```python
from build123d import *

# Parameters (mm, degrees)
SKETCH_1_W          = 280
SKETCH_1_H          = 60
EXTRUDE_1_DEPTH     = 4
HOLE_WIZARD_M4_1_D  = 3.3
SKETCH_10_W         = 3
SKETCH_10_H         = 60
EXTRUDE_4_DEPTH     = 95
EXTRUDE_8_DEPTH     = 60
SKETCH_14_W         = 75
SKETCH_14_H         = 45
EXTRUDE_10_DEPTH    = 10
SHELL_START         = -12
SHELL_1_OUTLINE_W   = 69
SHELL_1_OUTLINE_H   = 7
SHELL_1_DEPTH       = 42
SHELL_START_2       = -27
SHELL_1_2_DEPTH     = 15
CUT_EXTRUDE_2_REACH = 309.898
CUT_EXTRUDE_3_REACH = 184.211


# Read off the part's stored shape, not the designer's step: 抽壳1
with BuildPart() as part:
    # 草图1 → 凸台-拉伸1 (new body)
    with BuildSketch(Plane(origin=(0, 0, 0), x_dir=(0, 0, -1), z_dir=(1, 0, 0))):
        Rectangle(SKETCH_1_W, SKETCH_1_H)
    extrude(amount=EXTRUDE_1_DEPTH)

    # M4 螺纹孔1 (through all)
    with Locations(Plane(origin=(4, 20, -129), x_dir=(0, 0, 1), z_dir=(1, 0, 0))):
        with Locations((0, 0), (28, 0), (28, 40), (0, 40)):
            Hole(HOLE_WIZARD_M4_1_D / 2)

    # 草图10 → 凸台-拉伸4 (add)
    with BuildSketch(Plane(origin=(4, 0, 0), x_dir=(0, 0, -1), z_dir=(1, 0, 0))):
        with Locations((-138.5, 0)):
            Rectangle(SKETCH_10_W, SKETCH_10_H)
    extrude(amount=EXTRUDE_4_DEPTH)

    # 草图11 → 凸台-拉伸8 (add)
    with BuildSketch(Plane(origin=(0, 30, 0), x_dir=(1, 0, 0), z_dir=(0, 1, 0))):
        Polygon((4, -127), (14, -137), (4, -137), align=None)
    extrude(amount=-EXTRUDE_8_DEPTH)

    # 草图14 → 凸台-拉伸10 (add)
    with BuildSketch(Plane.XY.offset(140)):
        with Locations((61.5, 7.5)):
            Rectangle(SKETCH_14_W, SKETCH_14_H)
    extrude(amount=EXTRUDE_10_DEPTH)

    # 抽壳1 outline → 抽壳1 (cut)
    with BuildSketch(Plane(origin=(0, 0, 0), x_dir=(1, 0, 0), z_dir=(0, 1, 0)).offset(SHELL_START)):
        with Locations((61.5, -143.5)):
            Rectangle(SHELL_1_OUTLINE_W, SHELL_1_OUTLINE_H)
        Polygon((3, -137), (9.757359313, -137), (3, -130.242640687), align=None)
    extrude(amount=SHELL_1_DEPTH, mode=Mode.SUBTRACT)

    # Shell 1 2 outline → Shell 1 2 (cut)
    with BuildSketch(Plane(origin=(0, 0, 0), x_dir=(1, 0, 0), z_dir=(0, 1, 0)).offset(SHELL_START_2)):
        Polygon((3, -137), (9.757359313, -137), (3, -130.242640687), align=None)
    extrude(amount=SHELL_1_2_DEPTH, mode=Mode.SUBTRACT)

    # 切除-拉伸2: up to this face of the body (flat: up to its plane)
    cut_extrude_2_end = Plane(part.part.faces().sort_by_distance((56.5, 0, 137))[0])
    # 草图15 → 切除-拉伸2 (cut, up to the picked face)
    with BuildSketch(Plane.XY.offset(150), mode=Mode.PRIVATE) as cut_extrude_2_sk1:
        Polygon((61.5, 30), (29, 30), (29, 5), (44, -10), (61.5, -10), align=None)
    cut_extrude_2_tool1 = split(extrude(cut_extrude_2_sk1.sketch, amount=-CUT_EXTRUDE_2_REACH, mode=Mode.PRIVATE), bisect_by=cut_extrude_2_end, keep=Keep.BOTH, mode=Mode.PRIVATE)
    # 草图15 → 切除-拉伸2 (cut, up to the picked face)
    with BuildSketch(Plane.XY.offset(150), mode=Mode.PRIVATE) as cut_extrude_2_sk2:
        Polygon((94, 30), (61.5, 30), (61.5, -10), (79, -10), (94, 5), align=None)
    cut_extrude_2_tool2 = split(extrude(cut_extrude_2_sk2.sketch, amount=-CUT_EXTRUDE_2_REACH, mode=Mode.PRIVATE), bisect_by=cut_extrude_2_end, keep=Keep.BOTH, mode=Mode.PRIVATE)
    add(cut_extrude_2_tool1.solids().sort_by(Axis((46.315789, 11.421053, 150), (0, 0, -1)))[0], mode=Mode.SUBTRACT)
    add(cut_extrude_2_tool2.solids().sort_by(Axis((76.684211, 11.421053, 150), (0, 0, -1)))[0], mode=Mode.SUBTRACT)

    # 草图16 → 切除-拉伸3 (cut, up to next)
    with BuildSketch(Plane.ZY, mode=Mode.PRIVATE) as cut_extrude_3_sk1:
        with BuildLine():
            Line((-76, 24), (120, 24))
            ThreePointArc((120, 24), (127.071067812, 21.071067812), (130, 14))
            Line((130, 14), (130, -14))
            ThreePointArc((130, -14), (127.071067812, -21.071067812), (120, -24))
            Line((120, -24), (-76, -24))
            ThreePointArc((-76, -24), (-83.071067812, -21.071067812), (-86, -14))
            Line((-86, -14), (-86, 14))
            ThreePointArc((-86, 14), (-83.071067812, 21.071067812), (-76, 24))
        make_face()
    cut_extrude_3_tool1 = extrude(cut_extrude_3_sk1.sketch, amount=-CUT_EXTRUDE_3_REACH, mode=Mode.PRIVATE) & part.part
    add(cut_extrude_3_tool1.solids().sort_by_distance((0, 0, 22))[0], mode=Mode.SUBTRACT)


solid = part.part
```
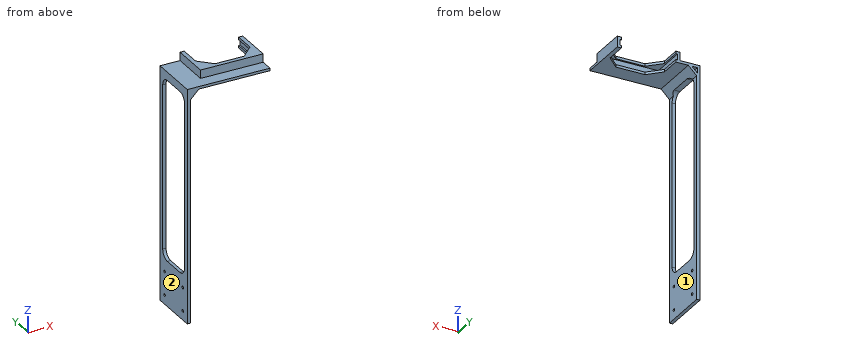
The listing builds one solid part. Answer for the finished solid, in the listing's coordinates (mm). Face numbers are marked on the shaded views. A direction names the side the tool comes from. Coordinates: 2 decimals unless noted, no trailing zeros. Loops run counter-clockwise (first coordinate to the right, second up) from the corner with the lowest first, then second, coordinate; pieces in that order, holes last. Notation, with made-up numbers: (64, 53.5) - (84, 53.5) arc R30 cw to (84, 76.5) - close; hole circle Ø6 at (-17.75, -10). An arc over 180 degrees is marked (long way). Write item = value, one per line.
1) Section C-C (x = 51.5) is taken. Determine the outline of the cut face in (y, z), plus the area to 3 significant figures.
Responses:
outline = (-30, 137) - (-10, 137) - (-10, 140) - (-12, 140) - (-12, 147) - (-10, 147) - (-10, 150) - (-15, 150) - (-15, 140) - (-30, 140) - close
area = 96.0 mm^2
2) Section B-B (z = -70) is taken. Determine the outline of the cut face in (x, y).
Responses:
outline = (0, -30) - (4, -30) - (4, -24) - (0, -24) - close; (0, 24) - (4, 24) - (4, 30) - (0, 30) - close
3) Find the intervals of material crossed by line 1 along Y through (x, z) = (2.55, -129); line 2 along Z through (x, y) = (1.5, -20); line 3 along Z through (x, y) = (29, -2), in increasing order.
Responses:
line_1 = -30 to -21.65, -18.35 to 18.35, 21.65 to 30
line_2 = -140 to -130.65, -127.35 to -102.65, -99.35 to -84, 128 to 140
line_3 = 137 to 140, 147 to 150
4) Each of these flat-tipped pins is pushed along its axis until it touches: P1, Ø5.5, axis at x = 7, z = 134.5, coming from the +Y side; P2, Ø0.9, axis at x = 54, z = 148, coming from the +Y side; P3, Ø8, axis at x = 72, z = 144.5, coming from the -Y side; P4, Ø5.5, axis at y = -4.5, z = 133.5, coming from the +X side. Where does it stop, or does it pass through?
Responses:
P1 = 30
P2 = -10
P3 = -15
P4 = 13.25
5) Section A-A (y = -5) is taken. Determine the outline of the cut face in (x, z).
Responses:
outline = (0, -140) - (4, -140) - (4, -86) - (0, -86) - close; (0, 130) - (7, 130) - (14, 137) - (39, 137) - (39, 140) - (27, 140) - (27, 147) - (39, 147) - (39, 150) - (24, 150) - (24, 140) - (0, 140) - close; (84, 137) - (99, 137) - (99, 150) - (84, 150) - (84, 147) - (96, 147) - (96, 140) - (84, 140) - close; hole (3, 130.24) - (9.76, 137) - (3, 137) - close
6) Which of the six approach directions +Z, -Z, +X, -X, +Y, -Y give full straight-line access (tool end or side, diameter ignored) to the marked faces 1 and 2?
Responses:
face_1 = -Z, +X, +Y, -Y
face_2 = +Z, -Z, -X, +Y, -Y
